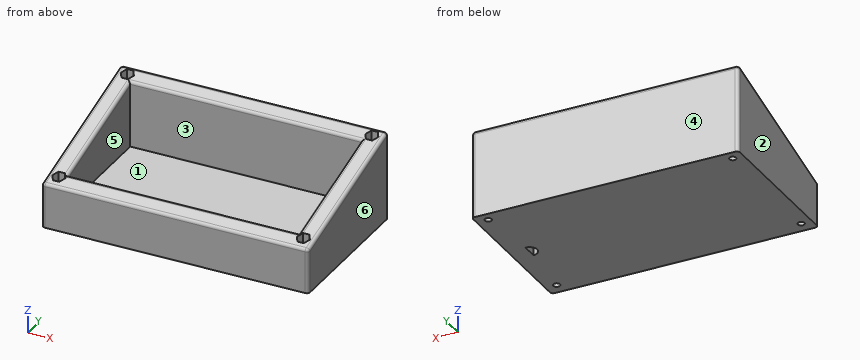
```python
from build123d import *

# Parameters (mm, degrees)
F0_W      = 120
F0_H      = 70
F1_DEPTH  = 40
F3_DEPTH  = 120.001
F4_T      = -8
F5_R      = 1.5
F8_DEPTH  = 35
F9_R      = 1.5
F10_DEPTH = 40.001
F12_DEPTH = 25


with BuildPart() as f1:
    # F0 (on Top) → F1 (new body)
    with BuildSketch(Plane.XY):
        with Locations((10.593040958, 9.0129598636)):
            Rectangle(F0_W, F0_H)
    extrude(amount=F1_DEPTH)

    # F2 (on face) → F3 (cut, through all)
    with BuildSketch(Plane(origin=(-49.406959042, 0, 0), x_dir=(0, -1, 0), z_dir=(-1, 0, 0))):
        Polygon((25.9870401364, 40), (-44.0129598636, 40), (25.9870401364, 20), align=None)
    extrude(amount=-F3_DEPTH, mode=Mode.SUBTRACT)

    # F4
    f4_openings = [f1.faces().sort_by_distance(p)[0] for p in [
        (10.593041, 9.01296, 30),
    ]]
    offset(amount=F4_T, openings=f4_openings)

    # F5
    f5_edges = [f1.edges().sort_by_distance(p)[0] for p in [
        (-49.406959, -25.98704, 10),
        (-49.406959, 44.01296, 20),
        (70.593041, 44.01296, 20),
        (70.593041, -25.98704, 10),
        (10.593041, 44.01296, 40),
        (70.593041, 9.01296, 30),
        (10.593041, -25.98704, 20),
        (-49.406959, 9.01296, 30),
        (10.593041, -17.98704, 22.285714),
        (62.593041, 9.01296, 30),
        (10.593041, 36.01296, 37.714286),
        (-41.406959, 9.01296, 30),
    ]]
    fillet(f5_edges, radius=F5_R)

    # F7 (on offset) → F8 (cut)
    with BuildSketch(Plane.XY.offset(40)):
        Polygon((-43.0277708034, 37.0129598636), (-41.5843951305, 39.5129598636), (-43.0277708034, 42.0129598636), (-45.9145221494, 42.0129598636), (-47.3578978224, 39.5129598636), (-45.9145221494, 37.0129598636), align=None)
        Polygon((66.9722291966, 37.0129598636), (68.4156048695, 39.5129598636), (66.9722291966, 42.0129598636), (64.0854778506, 42.0129598636), (62.6421021776, 39.5129598636), (64.0854778506, 37.0129598636), align=None)
        Polygon((-43.0277708034, -22.9870401364), (-41.5843951305, -20.4870401364), (-43.0277708034, -17.9870401364), (-45.9145221494, -17.9870401364), (-47.3578978224, -20.4870401364), (-45.9145221494, -22.9870401364), align=None)
        Polygon((66.9722291966, -22.9870401364), (68.4156048695, -20.4870401364), (66.9722291966, -17.9870401364), (64.0854778506, -17.9870401364), (62.6421021776, -20.4870401364), (64.0854778506, -22.9870401364), align=None)
    extrude(amount=-F8_DEPTH, mode=Mode.SUBTRACT)

    # F9 (on offset) → F10 (cut, through all)
    with BuildSketch(Plane.XY.offset(40)):
        with Locations((-44.5364899848, 39.5145639777)):
            Circle(F9_R)
        with Locations((65.4635100152, 39.5145639777)):
            Circle(F9_R)
        with Locations((65.4635100152, -20.4854360223)):
            Circle(F9_R)
        with Locations((-44.5364899848, -20.4854360223)):
            Circle(F9_R)
    extrude(amount=-F10_DEPTH, mode=Mode.SUBTRACT)

    # F11 (on face) → F12 (cut)
    with BuildSketch(Plane.XY.offset(8)):
        with BuildLine():
            Line((62.593040958, 5.5129598636), (62.593040958, 12.5129598636))
            ThreePointArc((62.593040958, 12.5129598636), (59.093040958, 9.0129598636), (62.593040958, 5.5129598636))
        make_face()
    extrude(amount=-F12_DEPTH, mode=Mode.SUBTRACT)


solid = f1.part
```
The listing builds one solid part. Answer for the finished solid, in the listing's coordinates (mm). Face numbers are marked on the shaded views. A direction names the side the tool comes from. Coordinates: 2 decimals unless noted, no trailing zeros. Write each loop counter-clockwise with the first axis right and the second up, starting at its lowest first coordinate (ties: lowest second). Pieces come first, ordered by that corner, then holes. Notation, with made-up numbers: (73, 30.25) -> (132, 30.25) arc R13 ccw to (132, 53.25) -> close; hole circle Ø4 at (26.5, 7.25). An arc over 180 degrees is marked (long way). Write each question's results on one line, items separated by ' | '. Start each with the question number.
1) A cutting plane is placed at B-B (x = 14.5). Determine the outline of the cut face in (y, z), then the cut area to 3 significant figures.
2) Straight lines are drawn through the part: probe 1 along Y at (x, z) = (46, 9); probe 2 along X at (y, z) = (11.5, 23); probe 3 along X at (y, z) = (41, 18). For each, find the intervals that lie inside material, in ascending order.
3) For a pull along Y with two mould halves and no side action, classify the marked faces 3, 4, 5 and 6 as +Y half, -Y half, draft (parallel to the pull), parting line (faces both ways), or undercut.
4) A tool of negligible diameter and unlimited length cuts with its end or side. For the marked faces 1 and 2, from which of +Z, -Z, +X, -X, +Y, -Y can it reach the whole face along a straight path? Write none if from no direction.
5) A cutting plane is placed at A-A (z = 11). Count the separate pieces of the cut face and the enclosed holes in it, then the cut area to 3 significant figures.
6) Flat-ended cylindrical pins translate along their axes: pin 1 Ø1.8 at (x, y) = (-44.54, 39.51) entering from +Z; pin 2 Ø2.5 at (x, y) = (64.5, -21.5) entering from +Z; pin 3 Ø3.5 at (x, y) = (65.46, 39.51) entering from -Z; pin 4 Ø3 at (x, z) = (66, 22.5) entering from -Y. Find the tip coordinate at first contact, or state that the pin passes through.
Values follow:
1) outline: (-25.99, 0) -> (44.01, 0) -> (44.01, 38.01) arc R1.5 ccw to (42.1, 39.45) -> (37.1, 38.03) arc R1.5 ccw to (36.01, 36.58) -> (36.01, 8) -> (-17.99, 8) -> (-17.99, 20.3) arc R1.5 ccw to (-19.9, 21.74) -> (-24.9, 20.31) arc R1.5 ccw to (-25.99, 18.87) -> close | area: 910 mm²
2) probe 1: -25.99 to -17.99, 36.01 to 44.01 | probe 2: -49.41 to -41.41, 62.59 to 70.59 | probe 3: -49.41 to -46.5, -42.44 to 63.5, 67.56 to 70.59
3) face 3: undercut | face 4: +Y half | face 5: undercut | face 6: draft
4) face 1: +Z | face 2: +Z, -Z, -X, +Y, -Y
5) separate pieces: 1 | enclosed holes: 5 | area: 2,700 mm²
6) pin 1: through | pin 2: z = 21.27 | pin 3: z = 0 | pin 4: y = -18.79
